```python
from build123d import *

# Parameters (mm, degrees)
F0_W      = 133.715108037
F0_H      = 59.3623146415
F1_DEPTH  = 3.5
F2_R      = 6.6440898667
F3_DEPTH  = 61.2
F4_R      = 4.997826556
F5_DEPTH  = 1.4
F6_R      = 7.6010927322
F7_DEPTH  = 1
F9_R      = 4.8490813771
F10_DEPTH = 1


# Not quite as in the source:
# - a fillet or chamfer that OpenCascade refuses, or shapes differently, is made with other operations: its cross-section is extruded or revolved along the edge and cut away or added


with BuildPart() as f1:
    # F0 (on Top) → F1 (new body)
    with BuildSketch(Plane.XY):
        Rectangle(F0_W, F0_H)
    extrude(amount=F1_DEPTH)

    # F2 (on face) → F3 (join)
    with BuildSketch(Plane(origin=(0, 0, 0), x_dir=(1, 0, 0), z_dir=(0, 0, -1))):
        with Locations((-58.0631382763, 21.2864857167)):
            Circle(F2_R)
        with Locations((-58.0631382763, -21.2864857167)):
            Circle(F2_R)
        with Locations((58.0631382763, 21.2864857167)):
            Circle(F2_R)
        with Locations((58.0631382763, -21.2864857167)):
            Circle(F2_R)
    extrude(amount=F3_DEPTH)

    # F4 (on face) → F5 (join)
    with BuildSketch(Plane.XY.offset(3.5)):
        with Locations((-53.4660555422, 0)):
            Circle(F4_R)
    extrude(amount=F5_DEPTH)

    # F6 (on face) → F7 (join)
    with BuildSketch(Plane.XY.offset(4.9)):
        with Locations((-53.4660555422, 0)):
            Circle(F6_R)
    extrude(amount=F7_DEPTH)

    # F8: fillet of radius 3.6213203436 on 1 edges, made by hand

    # F8_s1 → F8_t2 (revolve, cut)
    with BuildSketch(Plane.XZ):
        with BuildLine():
            ThreePointArc((-45.86496281, 5.9), (-47.0178827806, 5.1592821435), (-48.3634905139, 4.9))
            Line((-48.3634905139, 4.9), (-45.86496281, 4.9))
            Line((-45.86496281, 4.9), (-45.86496281, 5.9))
        make_face()
    revolve(axis=Axis((-53.4660555422, 0, 4.9), (0, 0, 1)), mode=Mode.SUBTRACT)

    # F9 (on face) → F10 (cut)
    with BuildSketch(Plane.XY.offset(5.9)):
        with Locations((-53.4660555422, 0)):
            Circle(F9_R)
    extrude(amount=-F10_DEPTH, mode=Mode.SUBTRACT)


solid = f1.part
```
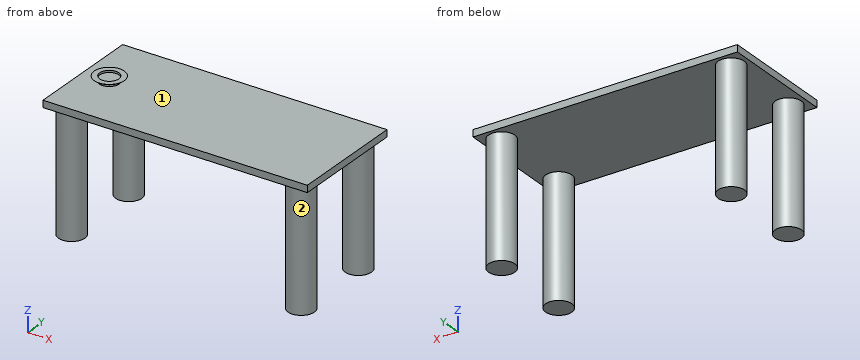
Design review of the part built by this model. Coordinates are the model's own, in mm. Face numbers are marked on the shaded views. Round coordinates to 2 decimals unless told otherwise and drop trailing zeros. Write each loop counter-clockwise with the first axis right and the second up, starting at its lowest first coordinate (ties: lowest second). Pieces come first, ordered by that corner, then holes. Notation, with made-up numbers: (60.5, -13) -> (81.5, -13) arc R23 cw to (81.5, 6) -> close; hole circle Ø5 at (-8, 85). An arc over 180 degrees is marked (long way). Answer in a Markdown table with one row per item.
Q1. To check wall thickness, follow L1, parallel to Z at x = -21.5, y = 25; L2, parallel to X at y = 19, z = -44; L3, parallel to X at y = 17.5, z = -15. State the ranges of each line that lie inside material, in increasing order. Write a range as [from, to].
The answers:
| item | result |
|---|---|
| L1 | [0, 3.5] |
| L2 | [-64.3, -51.82], [51.82, 64.3] |
| L3 | [-63.52, -52.6], [52.6, 63.52] |
Q2. Take a section at B-B, the plane z = -52. State the section outline as (x, y) points.
The answers:
| item | result |
|---|---|
| outline | circle Ø13.29 at (-58.06, -21.29); circle Ø13.29 at (-58.06, 21.29); circle Ø13.29 at (58.06, -21.29); circle Ø13.29 at (58.06, 21.29) |
Q3. Take a section at D-D, the plane y = -24. State the section outline as (x, z) points.
The answers:
| item | result |
|---|---|
| outline | (-66.86, 0) -> (-64.13, 0) -> (-64.13, -61.2) -> (-52, -61.2) -> (-52, 0) -> (52, 0) -> (52, -61.2) -> (64.13, -61.2) -> (64.13, 0) -> (66.86, 0) -> (66.86, 3.5) -> (-66.86, 3.5) -> close |
Q4. Draft analysis for pull direction X (two halves, no side actions). For the marked faces 1 and 2, state which applies: +X half, -X half, draft (parallel to the pull), parting line (faces both ways), or undercut.
The answers:
| item | result |
|---|---|
| face 1 | draft |
| face 2 | undercut |
Q5. Take a section at A-A, the plane y = 0. State the section outline as (x, z) points.
The answers:
| item | result |
|---|---|
| outline | (-66.86, 0) -> (66.86, 0) -> (66.86, 3.5) -> (-48.47, 3.5) -> (-48.47, 4.9) -> (-48.36, 4.9) arc R3.62 ccw to (-45.86, 5.9) -> (-48.62, 5.9) -> (-48.62, 4.9) -> (-58.32, 4.9) -> (-58.32, 5.9) -> (-61.07, 5.9) arc R3.62 ccw to (-58.57, 4.9) -> (-58.46, 4.9) -> (-58.46, 3.5) -> (-66.86, 3.5) -> close |
Q6. Clearance check with flat-ended pins moving along their axes: pin 1 Ø5 at (y, z) = (-20, -26) entering from +X; pin 2 Ø10 at (y, z) = (-5.5, -7.5) entering from -X; pin 3 Ø6 at (x, y) = (13.5, 5.5) entering from -Z; pin 4 Ø8 at (x, y) = (-53, -1.5) entering from +Z. State where each tip first meets the part, or that it passes through.
The answers:
| item | result |
|---|---|
| pin 1 | x = 64.71 |
| pin 2 | through |
| pin 3 | z = 0 |
| pin 4 | z = 5.9 |
Q7. Take a section at C-C, the plane x = 54. State the section outline as (y, z) points, then the cut area to 3 significant figures.
The answers:
| item | result |
|---|---|
| outline | (-29.68, 0) -> (-26.54, 0) -> (-26.54, -61.2) -> (-16.03, -61.2) -> (-16.03, 0) -> (16.03, 0) -> (16.03, -61.2) -> (26.54, -61.2) -> (26.54, 0) -> (29.68, 0) -> (29.68, 3.5) -> (-29.68, 3.5) -> close |
| area | 1,490 mm² |
